The listing builds one solid part. Answer for the finished solid, in the listing's coordinates (mm). Round coordinates to 2 decimals unless told otherwise and drop trailing zeros. Write each loop counter-clockwise with the first axis right and the second up, starting at its lowest first coordinate (ties: lowest second). Pieces come first, ordered by that corner, then holes. Notation, with made-up numbers: M 77.5,4.5 L 135.5,4.5 A17 ccw 135.5,11.5 Z; hole C 16.25,50.25 d7. An arc over 180 degrees is marked long. Put each result on its own line as item: value. Start each with the question number.
Autodesk Inventor part; units mm, degrees
ref_plane "YZ Plane" through (0, 0, 0) normal (1, 0, 0) x (0, 1, 0)
ref_plane "XZ Plane" through (0, 0, 0) normal (0, 1, 0) x (-1, 0, 0)
ref_plane "XY Plane" through (0, 0, 0) normal (0, 0, 1) x (1, 0, 0)
sketch "Sketch1" plane through (0, 0, 0) normal (0, 1, 0) x (-1, 0, 0)
  line L0 (55, -48) -> (-55, -48)
  line L1 (-60, -43) -> (-60, 43)
  line L2 (-55, 48) -> (55, 48)
  line L3 (60, 43) -> (60, -43)
  line L4 (50, -35) -> (-50, -35) construction
  line L5 (-50, -35) -> (-50, 35) construction
  line L6 (-50, 35) -> (50, 35) construction
  line L7 (50, 35) -> (50, -35) construction
  arc A0 (60, 43) -> (55, 48) centre (55, 43) ccw
  arc A1 (-55, 48) -> (-60, 43) centre (-55, 43) ccw
  arc A2 (-60, -43) -> (-55, -48) centre (-55, -43) ccw
  arc A3 (55, -48) -> (60, -43) centre (55, -43) ccw
  circle A4 centre (50, -35) radius 3.4
  circle A5 centre (50, 35) radius 3.4
  circle A6 centre (-50, -35) radius 3.4
  circle A7 centre (-50, 35) radius 3.4
  line L8 (0, -20) -> (0, 20) construction
  line L9 (25, -20) -> (25, 20) construction
  line L10 (-25, 20) -> (-25, -20) construction
  arc A8 (-25, -20) -> (25, -20) centre (0, -20) ccw construction
  arc A9 (25, 20) -> (-25, 20) centre (0, 20) ccw construction
  circle A10 centre (0, -20) radius 21.25 construction
  circle A11 centre (-21.25, -20) radius 2
  circle A12 centre (-10.625, -38.403) radius 2
  circle A13 centre (10.625, -38.403) radius 2
  circle A14 centre (21.25, -20) radius 2
  circle A15 centre (10.625, -1.597) radius 2
  circle A16 centre (-10.625, -1.597) radius 2
  point P0 (0, 0)
  point P1 (-60, 0)
  point P2 (0, -48)
  point P3 (0, -35)
  point P4 (-50, 0)
  point P5 (0, 0)
  dimension "d17" = 42.5
  dimension "d0" = 96
  dimension "d1" = 120
  dimension "d2" = 70
  dimension "d3" = 100
  dimension "d4" = 5
  dimension "d5" = 6.8
  dimension "d6" = 6.8
  dimension "d8" = 6.8
  dimension "d10" = 6.8
  dimension "d13" = 25
  dimension "d14" = 40
  dimension "d23" = 4
  dimension "d26" = 360
extrude "Extrusion1" add sketch "Sketch1" along normal blind 6
equation "\"d17\" = iciclesMountD"
equation "\"d0\" = moduleHeight"
equation "\"d1\" = moduleWidth"
equation "\"d2\" = moduleMountH"
equation "\"d3\" = moduleMountW"
equation "\"d4\" = moduleCornerR"
equation "\"d5\" = moduleMountD"
equation "\"d6\" = moduleMountD"
equation "\"d8\" = moduleMountD"
equation "\"d10\" = moduleMountD"
equation "\"d13\" = moduleOpeningR"
equation "\"d14\" = moduleOpeningH"
equation "\"d23\" = insertDrillM3"
equation "\"d15\" = thickness"
equation "\"moduleWidth\" = 120"
equation "\"moduleHeight\" = 96"
equation "\"moduleMountW\" = 100"
equation "\"moduleMountH\" = 70"
equation "\"moduleMountD\" = 6.8"
equation "\"moduleCornerR\" = 5"
equation "\"moduleOpeningR\" = 25"
equation "\"moduleOpeningH\" = 40"
equation "\"thickness\" = 6"
equation "\"iciclesMountD\" = 42.5"
equation "\"insertDrillM3\" = 4"
properties part number "Module_base_Icicles26"
Item 1: Section C-C (x = -50) is taken. Give the vertices of the cut face in (y, z).
Item 2: Section D-D (y = 1.3) is taken. Count the separate pieces of the cut face and the enclosed holes in it, and give its area (3 significant figures).
Item 3: A flat-ended cylindrical pin translates along its axis: pin 1 (5.5 mm diameter, centred on x = 50, z = 35, fed in from +Y). Find the tip coordinate at first contact, or state that the pin passes through.
Item 4: Determine the mould class of faces 1 (the cylindrical face through (59, 3, 46)), 2 (the cylindrical face through (12.1, 2.96, -2.95)), 3 (the flat face through (1, 6, 1)) for opening direction X: released by +X, released by -X, zero draft, split by the parting line, or undercut.
Item 5: Section A-A (x = 21.25) is taken. Give the vertices of the cut face in (y, z).
Item 6: Consider line 1 along Z through (x, y) = (50, 1.35); line 2 along Z through (x, y) = (-52.5, 1.2); line 3 along X through (y, z) = (5.1, -37.5). Determine where each line is inside the solid, lowest interval first. Write a range as [from, to].
Item 7: Section B-B (z = -20) is taken. Give the vertices of the cut face in (x, y).
Output values:
1. outline: M 0,-48 L 6,-48 L 6,-38.4 L 0,-38.4 Z; M 0,-31.6 L 6,-31.6 L 6,31.6 L 0,31.6 Z; M 0,38.4 L 6,38.4 L 6,48 L 0,48 Z
2. separate pieces: 1
2. enclosed holes: 10
2. area: 11,300 mm^2
3. pin 1: passes through
4. face 1: released by +X
4. face 2: undercut
4. face 3: zero draft
5. outline: M 0,-48 L 6,-48 L 6,-22 L 0,-22 Z; M 0,-18 L 6,-18 L 6,48 L 0,48 Z
6. line 1: z = [-48, -38.4], [-31.6, 31.6], [38.4, 48]
6. line 2: z = [-48, -37.3], [-32.7, 32.7], [37.3, 48]
6. line 3: x = [-60, -52.3], [-47.7, -12.41], [-8.84, 8.84], [12.41, 47.7], [52.3, 60]
7. outline: M -60,0 L -23.25,0 L -23.25,6 L -60,6 Z; M -19.25,0 L 19.25,0 L 19.25,6 L -19.25,6 Z; M 23.25,0 L 60,0 L 60,6 L 23.25,6 Z
